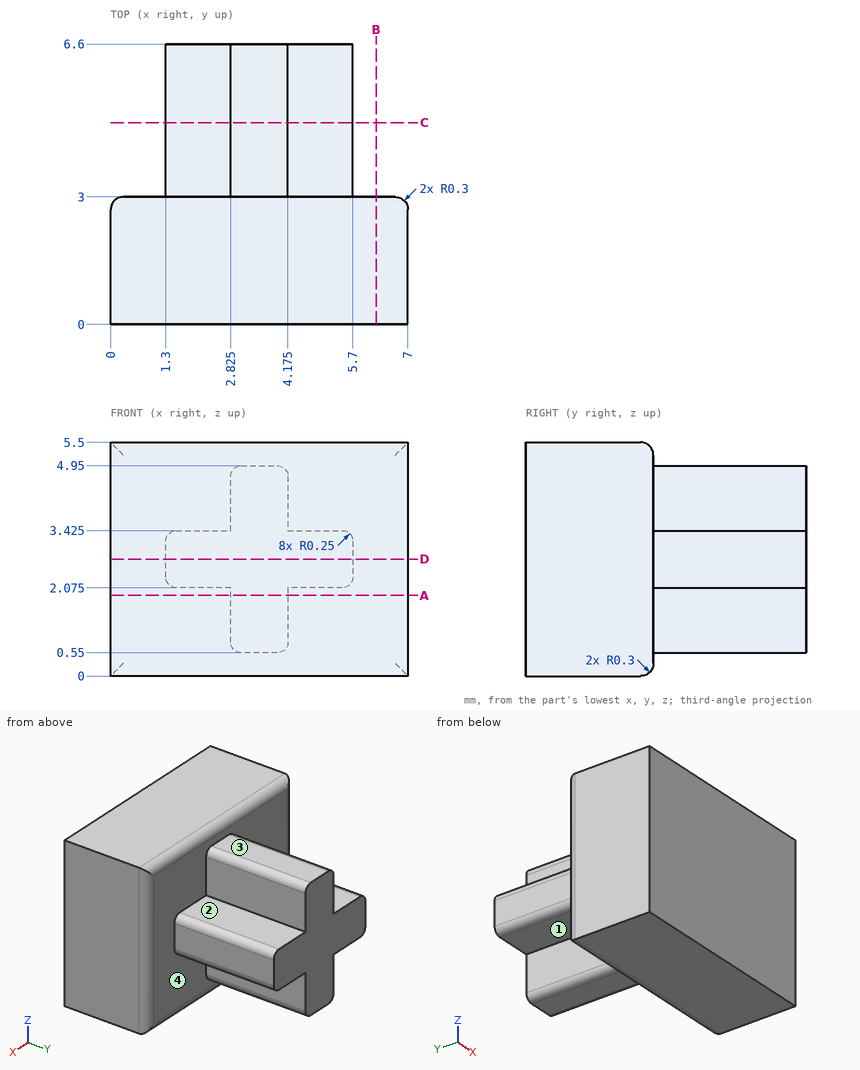
Geometry check sheet. Reference: drawing and pictorial views, mm from the part's lowest x, y, z. A direction names the side the tool comes from. Give positions to 0.01 mm unless a question says otherwise; leave off trailing zeros. Write each loop counter-clockwise with the first axis right and the second up, starting at its lowest first coordinate (ties: lowest second). Pieces come first, ordered by that corner, then holes. Notation, with made-up numbers: (2.25, 20) -> (17.25, 20) arc R20 cw to (17.25, 51) -> close; hole circle Ø4 at (28, 44). An arc over 180 degrees is marked (long way). One line per question, with ' | ' between items.
Item 1: Sectioned sample at C-C, the plane y = 4.75. Record the boundary of the cut face in (x, z) (3 decimals).
Determined:
outline: (1.3, 2.325) arc R0.25 ccw to (1.55, 2.075) -> (2.825, 2.075) -> (2.825, 0.8) arc R0.25 ccw to (3.075, 0.55) -> (3.925, 0.55) arc R0.25 ccw to (4.175, 0.8) -> (4.175, 2.075) -> (5.45, 2.075) arc R0.25 ccw to (5.7, 2.325) -> (5.7, 3.175) arc R0.25 ccw to (5.45, 3.425) -> (4.175, 3.425) -> (4.175, 4.7) arc R0.25 ccw to (3.925, 4.95) -> (3.075, 4.95) arc R0.25 ccw to (2.825, 4.7) -> (2.825, 3.425) -> (1.55, 3.425) arc R0.25 ccw to (1.3, 3.175) -> close
Item 2: Access from +Z, -Z, +X, -X, +Y, -Y to the whole of each face (thin tool, end or side, straight path). Record for the marked faces 1, 2, 3 and 4.
Determined:
face 1: -Z, -X, +Y | face 2: +Z, +X, +Y | face 3: +Z, +X, -X, +Y | face 4: +Y
Item 3: Sectioned sample at D-D, the plane z = 2.75. Record the boundary of the cut face in (x, y), plus the area to 3 significant figures.
Determined:
outline: (0, 0) -> (7, 0) -> (7, 2.7) arc R0.3 ccw to (6.7, 3) -> (5.7, 3) -> (5.7, 6.6) -> (1.3, 6.6) -> (1.3, 3) -> (0.3, 3) arc R0.3 ccw to (0, 2.7) -> close | area: 36.8 mm^2
Item 4: Depth check by flat-ended pin: pin 1 (1.4 mm diameter, centred on y = 5, z = 4, fed in from -X); pin 2 (1.4 mm diameter, centred on x = 2.5, y = 4.5, fed in from +Z); pin 3 (0.9 mm diameter, centred on y = 4, z = 3, fed in from +X); pin 4 (1 mm diameter, centred on x = 6.5, y = 5, fed in from -Z). Enter the tip coordinate at first touch or a pass-through.
Determined:
pin 1: x = 1.33 | pin 2: z = 4.95 | pin 3: x = 5.7 | pin 4: through
Item 5: Scan lines: line 1 along Y through (x, z) = (4.75, 5.05); line 2 along X through (y, z) = (5.25, 2) (3 decimals); line 3 along Z through (x, y) = (3.75, 5). Record each from-to range of solid material in increasing order.
Determined:
line 1: 0 to 3 | line 2: 2.825 to 4.175 | line 3: 0.55 to 4.95
Item 6: Sectioned sample at B-B, the plane x = 6.25. Record the boundary of the cut face in (y, z), plus the area to 3 significant figures.
Determined:
outline: (0, 0) -> (2.7, 0) arc R0.3 ccw to (3, 0.3) -> (3, 5.2) arc R0.3 ccw to (2.7, 5.5) -> (0, 5.5) -> close | area: 16.5 mm^2
Item 7: Sectioned sample at A-A, the plane z = 1.9. Record the boundary of the cut face in (x, y) (3 decimals), plus the area to 3 significant figures.
Determined:
outline: (0, 0) -> (7, 0) -> (7, 2.7) arc R0.3 ccw to (6.7, 3) -> (4.175, 3) -> (4.175, 6.6) -> (2.825, 6.6) -> (2.825, 3) -> (0.3, 3) arc R0.3 ccw to (0, 2.7) -> close | area: 25.8 mm^2
